Build history of the part. All positions in model axes, mm. Face numbers are marked on the shaded views. A direction names the side the tool comes from. Give positions to 0.01 mm unless a question says otherwise; leave off trailing zeros. Loops run counter-clockwise (first coordinate to the right, second up) from the corner with the lowest first, then second, coordinate; pieces in that order, holes last. Notation, with made-up numbers: M 35.5,-37.5 L 49.5,-37.5 A15 cw 49.5,-25.5 Z; hole C 20,75.5 d1. An arc over 180 degrees is marked long. Answer in a Markdown table with one row per item. Add a question column.
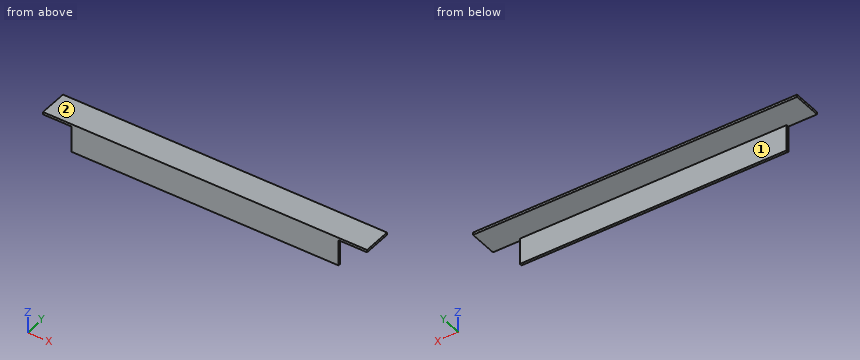
```python
from build123d import *

# Parameters (mm, degrees)
BOSS_EXTRUDE1_DEPTH = 215.9
CUT_EXTRUDE1_REACH  = 218.811
SKETCH2_W           = 19.05
SKETCH2_H           = 17.4244


with BuildPart() as part:
    # Sketch1 → Boss-Extrude1 (new body)
    with BuildSketch(Plane(origin=(0, 0, 0), x_dir=(0, 0, -1), z_dir=(1, 0, 0))):
        Polygon((-7.8994, -7.8994), (9.525, -7.8994), (9.525, -9.525), (-9.525, -9.525), (-9.525, 9.525), (-7.8994, 9.525), align=None)
    extrude(amount=BOSS_EXTRUDE1_DEPTH)

    # Sketch2 → Cut-Extrude1 (cut, up to next)
    with BuildSketch(Plane(origin=(0, -7.8994, 0), x_dir=(1, 0, 0), z_dir=(0, 1, 0)), mode=Mode.PRIVATE) as cut_extrude1_sk1:
        with Locations((9.525, 0.8128)):
            Rectangle(SKETCH2_W, SKETCH2_H)
    cut_extrude1_tool1 = extrude(cut_extrude1_sk1.sketch, amount=-CUT_EXTRUDE1_REACH, mode=Mode.PRIVATE) & part.part
    # Sketch2 → Cut-Extrude1 (cut, up to next)
    with BuildSketch(Plane(origin=(0, -7.8994, 0), x_dir=(1, 0, 0), z_dir=(0, 1, 0)), mode=Mode.PRIVATE) as cut_extrude1_sk2:
        with Locations((206.375, 0.8128)):
            Rectangle(SKETCH2_W, SKETCH2_H)
    cut_extrude1_tool2 = extrude(cut_extrude1_sk2.sketch, amount=-CUT_EXTRUDE1_REACH, mode=Mode.PRIVATE) & part.part
    add(cut_extrude1_tool1.solids().sort_by_distance((9.525, -7.8994, -0.8128))[0], mode=Mode.SUBTRACT)
    add(cut_extrude1_tool2.solids().sort_by_distance((206.375, -7.8994, -0.8128))[0], mode=Mode.SUBTRACT)


solid = part.part
```
(1) Tool access for the marked faces 1 and 2: list every direction of +Z, -Z, +X, -X, +Y, -Y with a clear straight run to the whole face (end or side of a thin tool).
(2) Slice it at A-A, the plane x = 84. Give the cut face in (y, z) (3 decimals).
(3) Pin check, flat tips, straight feed: pin 1 (3 mm diameter, centred on x = 118, y = -0.5, fed in from -Z); pin 2 (6 mm diameter, centred on x = 172, z = -2.5, fed in from +Y); pin 3 (0.8 mm diameter, centred on y = -8.5, z = -1.5, fed in from +X). Stop position of each tip, or through.
(4) Slice it at B-B, the plane z = -5.75. Give the cut face in (x, y) (3 decimals).
(5) Slice it at C-C, the plane y = -1.75. Give the cut face in (x, z) (3 decimals), then the cut area to 3 significant figures.
(6) Wall check: line 1 (Y direction, x = 54, z = 3.25) (3 decimals); line 2 (Z direction, x = 144, y = 3.25) (3 decimals); line 3 (X direction, y = -8, z = 1.75). Give the ranges that are in metal, low to high.
Solution:
| question | item | result |
|---|---|---|
| 1 | face 1 | -Z, +X, -X, +Y |
| 1 | face 2 | +Z, +X, -X, +Y, -Y |
| 2 | outline | M -9.525,-9.525 L -7.899,-9.525 L -7.899,7.899 L 9.525,7.899 L 9.525,9.525 L -9.525,9.525 Z |
| 3 | pin 1 | z = 7.9 |
| 3 | pin 2 | y = -7.9 |
| 3 | pin 3 | x = 196.85 |
| 4 | outline | M 19.05,-9.525 L 196.85,-9.525 L 196.85,-7.899 L 19.05,-7.899 Z |
| 5 | outline | M 0,7.899 L 215.9,7.899 L 215.9,9.525 L 0,9.525 Z |
| 5 | area | 351 mm^2 |
| 6 | line 1 | -9.525 to -7.899 |
| 6 | line 2 | 7.899 to 9.525 |
| 6 | line 3 | 19.05 to 196.85 |
